Read the model definition and answer for the solid it produces. Units are mm, in the model's axes. A direction names the side the tool comes from. Coordinates: 2 decimals unless noted, no trailing zeros. Order: outer loops, then holes, each group sorted by start corner. A loop starts at its lowest first (then second) coordinate and runs counter-clockwise, first axis right, second up. Notation, with made-up numbers: (-14, -5.75) - (-8, -5.75) arc R28 ccw to (-8, 23.25) - close; hole circle Ø6 at (61.5, 48.5). An arc over 180 degrees is marked (long way). Use one line per item in the form item = value.
```python
from build123d import *

# Parameters (mm, degrees)
BOSS_EXTRUDE1_DEPTH = 10
SKETCH2_R           = 5
SKETCH2_W           = 20
SKETCH2_H           = 20
BOSS_EXTRUDE2_DEPTH = 175
SKETCH3_R           = 5
BOSS_EXTRUDE3_DEPTH = 260
SKETCH4_R           = 5
SKETCH5_W           = 30
SKETCH5_H           = 20
CUT_EXTRUDE1_DEPTH  = 20
BOSS_EXTRUDE4_DEPTH = 2
SKETCH7_R           = 10
CUT_EXTRUDE2_DEPTH  = 30
SKETCH8_W           = 20
SKETCH8_H           = 290
BOSS_EXTRUDE5_DEPTH = 75.92
CUT_EXTRUDE3_DEPTH  = 290
SKETCH10_W          = 250
SKETCH10_H          = 47.150724805
CUT_EXTRUDE4_DEPTH  = 20


with BuildPart() as part:
    # Sketch1 → Boss-Extrude1 (new, symmetric)
    with BuildSketch(Plane(origin=(0, 0, 0), x_dir=(1, 0, 0), z_dir=(0, 1, 0))):
        Polygon((-330, 192.5), (50, 192.5), (130, 145), (330, 145), (330, 125), (330, -125), (330, -145), (130, -145), (50, -192.5), (-330, -192.5), (-330, -172.5), (44.50990723, -172.5), (124.50990723, -125), (310, -125), (310, 125), (124.50990723, 125), (44.50990723, 172.5), (-330, 172.5), align=None)
    extrude(amount=BOSS_EXTRUDE1_DEPTH, both=True)

    # Sketch2 → Boss-Extrude2 (add, symmetric)
    with BuildSketch(Plane.XY):
        with Locations(Location((-315, 0, 0), (0, 0, 180))):
            Circle(SKETCH2_R)
        with Locations((-230, 0)):
            Rectangle(SKETCH2_W, SKETCH2_H)
        with Locations((165, 0)):
            Rectangle(SKETCH2_W, SKETCH2_H)
    extrude(amount=BOSS_EXTRUDE2_DEPTH, both=True)

    # Sketch3 → Boss-Extrude3 (add, symmetric)
    with BuildSketch(Plane.XY):
        with Locations((-270, 0)):
            Circle(SKETCH3_R)
    extrude(amount=BOSS_EXTRUDE3_DEPTH, both=True)

    # Sweep1: sweep along a curve in space
    with BuildLine() as sweep1_path:
        Line((-95, -10, 182.5), (-95, -20, 182.5))
        ThreePointArc((-95, -20, 182.5), (-95, -27.071067812, 185.428932188), (-95, -30, 192.5))
        Line((-95, -30, 192.5), (-95, -30, 260))
    # Sketch4 → Sweep1 (sweep)
    with BuildSketch(Plane.XZ.offset(10)):
        with Locations((-95, 182.5)):
            Circle(SKETCH4_R)
        with Locations((45, 182.5)):
            Circle(SKETCH4_R)
    sweep1 = sweep(path=sweep1_path.line)

    # Mirror1: Sweep1 across plane
    add(sweep1.mirror(Plane.XY))

    # Sketch5 → Cut-Extrude1 (cut)
    with BuildSketch(Plane(origin=(175, 0, 0), x_dir=(0, 0, -1), z_dir=(1, 0, 0))):
        with Locations((-160, 0)):
            Rectangle(SKETCH5_W, SKETCH5_H)
        with Locations((160, 0)):
            Rectangle(SKETCH5_W, SKETCH5_H)
    extrude(amount=-CUT_EXTRUDE1_DEPTH, mode=Mode.SUBTRACT)

    # Sketch6 → Boss-Extrude4 (add)
    with BuildSketch(Plane(origin=(0, 10, 0), x_dir=(1, 0, 0), z_dir=(0, 1, 0))):
        Polygon((-220, -172.5), (-220, 172.5), (44.50990723, 172.5), (124.50990723, 125), (155, 125), (155, -125), (124.50990723, -125), (44.50990723, -172.5), align=None)
    extrude(amount=-BOSS_EXTRUDE4_DEPTH)

    # Sketch7 → Cut-Extrude2 (cut)
    with BuildSketch(Plane(origin=(0, 10, 0), x_dir=(1, 0, 0), z_dir=(0, 1, 0))):
        with Locations(Location((-190, 0, 0), (0, 0, 270))):
            Circle(SKETCH7_R)
    extrude(amount=-CUT_EXTRUDE2_DEPTH, mode=Mode.SUBTRACT)

    # Sketch8 → Boss-Extrude5 (add)
    with BuildSketch(Plane(origin=(0, 10, 0), x_dir=(1, 0, 0), z_dir=(0, 1, 0))):
        with Locations((166.85, 0)):
            Rectangle(SKETCH8_W, SKETCH8_H)
    extrude(amount=BOSS_EXTRUDE5_DEPTH)

    # Sketch9 → Cut-Extrude3 (cut)
    with BuildSketch(Plane.XY.offset(145)):
        Polygon((156.85, 85.92), (330, 10), (176.85, 85.92), align=None)
    extrude(amount=-CUT_EXTRUDE3_DEPTH, mode=Mode.SUBTRACT)

    # Sketch10 → Cut-Extrude4 (cut)
    with BuildSketch(Plane(origin=(176.85, 0, 0), x_dir=(0, 0, -1), z_dir=(1, 0, 0))):
        with Locations((0, 33.575362403)):
            Rectangle(SKETCH10_W, SKETCH10_H)
    extrude(amount=-CUT_EXTRUDE4_DEPTH, mode=Mode.SUBTRACT)


solid = part.part
```
(1) Section B-B, the plane y = 34 is taken. Write down the section's boundary in (x, z), then the cut area to 3 significant figures.
Answer list:
outline = (156.85, -145) - (176.85, -145) - (176.85, -125) - (156.85, -125) - close; (156.85, 125) - (176.85, 125) - (176.85, 145) - (156.85, 145) - close
area = 800 mm2
(2) Given pin 1 Ø9 at (x, y) = (136.5, 0.5) entering from -Z; pin 2 Ø14.5 at (x, y) = (142.5, 3.5) entering from +Z; pin 3 Ø6 at (x, z) = (168.5, -6) entering from -Y, each flat-ended and moving along its own axis, determine where each tip first touches the part or whether it passes through.
Answer list:
pin_1 = -145
pin_2 = 145
pin_3 = -10
(3) Section D-D, the plane x = -37 is taken. Write down the section's boundary in (y, z), then the cut area to 3 significant figures.
Answer list:
outline = (-10, -192.5) - (10, -192.5) - (10, 192.5) - (-10, 192.5) - (-10, 172.5) - (8, 172.5) - (8, -172.5) - (-10, -172.5) - close
area = 1,490 mm2
(4) Straight lines are drawn through the part: L1, parallel to X at y = 9, z = 0; L2, parallel to Z at x = 2, y = -2; L3, parallel to Y at x = 37, z = 75. For each, find the intervals that lie inside material, in ascending order.
Answer list:
L1 = -240 to -200, -180 to 175, 310 to 330
L2 = -192.5 to -172.5, 172.5 to 192.5
L3 = 8 to 10
(5) Section A-A, the plane z = -37 is taken. Write down the section's boundary in (x, y).
Answer list:
outline = circle Ø10 at (-315, 0); circle Ø10 at (-270, 0); (-240, -10) - (-220, -10) - (-220, 8) - (155, 8) - (155, -10) - (175, -10) - (175, 10) - (-240, 10) - close; (156.85, 57.15) - (176.85, 57.15) - (176.85, 77.15) - (156.85, 85.92) - close; (310, -10) - (330, -10) - (330, 10) - (310, 10) - close
(6) Section C-C, the plane z = -214 is taken. Write down the section's boundary in (x, y).
Answer list:
outline = circle Ø10 at (-270, 0); circle Ø10 at (-95, -30); circle Ø10 at (45, -30)
(7) Which of the six approach directions +Z, -Z, +X, -X, +Y, -Y give full straight-line access (tool end or side, diameter ignored) to faces 5 (the flat face through (83.95, -0.874, 149.082)), 6 (the flat face through (167, 57.151, 2)), 7 (the flat face through (311, 10, 10))?
Answer list:
face_5 = -Y
face_6 = +X, -X
face_7 = +Z, -Z, +X, +Y
(8) The mould has two halves that part along X. Classify faces 1 (the flat face through (176.85, 58, 2)), 2 (the flat face through (-330, 0, -182)), 3 (the flat face through (234, 8, 125)), 4 (the flat face through (-86, -1, -172.5)): +X half, -X half, draft (parallel to the pull), parting line (faces both ways), or undercut.
Answer list:
face_1 = +X half
face_2 = -X half
face_3 = undercut
face_4 = undercut
